from build123d import *

# Parameters (mm, degrees)
F1_DEPTH = 6
F3_DEPTH = 25


with BuildPart() as f1:
    # F0 (on Top) → F1 (new body)
    with BuildSketch(Plane.XY):
        Polygon((275, -50), (275, 50), (-275, 50), (-275, -50), (0, 0), align=None)
    extrude(amount=F1_DEPTH)

    # F2 (on face) → F3 (cut)
    with BuildSketch(Plane.XY.offset(6)):
        Polygon((-223.195529, -25.335087), (-260, 5.431539), (-260, -32.026809), align=None)
        Polygon((-202.192262, 29.317927), (-260, 25.445178), (-202.192262, -25.335087), align=None)
    extrude(amount=-F3_DEPTH, mode=Mode.SUBTRACT)


solid = f1.part
For this review, take the finished solid that the model builds, in its own axes (mm). A direction names the side the tool comes from. Round coordinates to 2 decimals unless told otherwise and drop trailing zeros. Write each loop counter-clockwise with the first axis right and the second up, starting at its lowest first coordinate (ties: lowest second). Pieces come first, ordered by that corner, then holes. Notation, with made-up numbers: M 83.25,-31.75 L 112.25,-31.75 A14 cw 112.25,-10.75 Z; hole C -17,16 d2. An arc over 180 degrees is marked long. Write item = value, one per line. Start each with the question number.
(1) We need section A-A (y = -36.5). Give the boundary of the cut face in (x, z).
(2) We need section B-B (z = 3.75). Give the boundary of the cut face in (x, y).
(3) We need section D-D (y = 11). Give the boundary of the cut face in (x, z), then the cut area to 3 significant figures.
(4) The part is to be moulded in two halves that separate along X. For faces 1 (the face through (-231.5, 0.41, 3.04)), 2 (the face through (-4, 12, 0)), say which applies: +X half, -X half, draft (parallel to the pull), parting line (faces both ways), or undercut.
(5) For line 1 along X through (y, z) = (5, 5); line 2 along X through (y, z) = (6.5, 1); line 3 along X through (y, z) = (24, 0.5), list the stretches that pass through material, from the lowest coordinate up.
(6) Clearance check with a flat-ended pin moving along its axis: pin 1 Ø1.5 at (x, z) = (-5.5, 4.5) entering from -Y. State where the tip first meets the part, or that it passes through.
(7) For faces 3 (the face through (-241.3, -10.2, 3)), 4 (the face through (-4, 12, 6)), 5 (the face through (135.58, -24.65, 2.96)), list the 3-axis set-ups (+Z, -Z, +X, -X, +Y, -Y) from which the entire face can be reached by the end or side of a thin tool; tool diameter is ignored.
(8) We need section C-C (y = -14.5). Give the boundary of the cut face in (x, z), then the cut area to 3 significant figures.
Results found:
q1.outline = M -275,0 L -200.75,0 L -200.75,6 L -275,6 Z; M 200.75,0 L 275,0 L 275,6 L 200.75,6 Z
q2.outline = M -275,-50 L 0,0 L 275,-50 L 275,50 L -275,50 Z; hole M -260,-32.03 L -223.2,-25.34 L -260,5.43 Z; hole M -260,25.45 L -202.19,-25.34 L -202.19,29.32 Z
q3.outline = M -275,0 L -243.56,0 L -243.56,6 L -275,6 Z; M -202.19,0 L 275,0 L 275,6 L -202.19,6 Z
q3.area = 3,050 mm²
q4.face_1 = undercut
q4.face_2 = draft
q5.line_1 = -275 to -260, -259.48 to -236.73, -202.19 to 275
q5.line_2 = -275 to -238.43, -202.19 to 275
q5.line_3 = -275 to -258.35, -202.19 to 275
q6.pin_1 = -1.14
q7.face_3 = +Z, -Z
q7.face_4 = +Z, +X, -X, +Y, -Y
q7.face_5 = +Z, -Z, -Y
q8.outline = M -275,0 L -260,0 L -260,6 L -275,6 Z; M -236.16,0 L -214.53,0 L -214.53,6 L -236.16,6 Z; M -202.19,0 L -79.75,0 L -79.75,6 L -202.19,6 Z; M 79.75,0 L 275,0 L 275,6 L 79.75,6 Z
q8.area = 2,130 mm²
